from build123d import *

# Parameters (mm, degrees)
F1_DEPTH = 10
F2_R     = 11
F3_DEPTH = 7.5
F4_R     = 4
F5_DEPTH = 7
F6_R     = 5
F7_DEPTH = 25
F8_R     = 2


# Not quite as in the source:
# - a feature names something its author has since deleted; it is built from what else it names


with BuildPart() as f1:
    # F0 (on Top) → F1 (new body)
    with BuildSketch(Plane.XY):
        with BuildLine():
            Line((29.69714, -15), (29.69714, 0))
            ThreePointArc((29.69714, 0), (27.1937406538, 6.0437406538), (21.15, 8.54714))
            Line((21.15, 8.54714), (12.3266539588, 8.54714))
            ThreePointArc((12.3266539588, 8.54714), (0, 15), (-12.3266539588, 8.54714))
            Line((-12.3266539588, 8.54714), (-21.15, 8.54714))
            ThreePointArc((-21.15, 8.54714), (-29.69714, 0), (-21.15, -8.54714))
            Line((-21.15, -8.54714), (-12.3266539588, -8.54714))
            ThreePointArc((-12.3266539588, -8.54714), (-6.9567557094, -13.2892268398), (0, -15))
            Line((0, -15), (29.69714, -15))
        make_face()
    extrude(amount=F1_DEPTH)

    # F2 (on face) → F3 (cut)
    with BuildSketch(Plane.XY.offset(10)):
        Circle(F2_R)
    extrude(amount=-F3_DEPTH, mode=Mode.SUBTRACT)

    # F4 (on face) → F5 (cut)
    with BuildSketch(Plane(origin=(0, 0, 0), x_dir=(1, 0, 0), z_dir=(0, 0, -1))):
        with Locations((-21.15, 0)):
            Circle(F4_R)
        with Locations((21.15, 0)):
            Circle(F4_R)
    extrude(amount=-F5_DEPTH, mode=Mode.SUBTRACT)

    # F6 (on face) → F7 (cut)
    with BuildSketch(Plane.XY.offset(2.5)):
        with Locations((0, 0.6768586167)):
            Circle(F6_R)
    extrude(amount=-F7_DEPTH, mode=Mode.SUBTRACT)

    # F8
    f8_edges = [f1.edges().sort_by_distance(p)[0] for p in [
        (29.69714, -15, 5),
    ]]
    fillet(f8_edges, radius=F8_R)


solid = f1.part
Here's how the part is built. I have some questions about the finished solid (model axes, mm). A direction names the side the tool comes from. Give positions to 0.01 mm unless a question says otherwise; leave off trailing zeros. Write each loop counter-clockwise with the first axis right and the second up, starting at its lowest first coordinate (ties: lowest second). Pieces come first, ordered by that corner, then holes. Notation, with made-up numbers: (59.5, 37.25) -> (75.5, 37.25) arc R3 ccw to (75.5, 41.25) -> close; hole circle Ø10 at (-11, -16). An arc over 180 degrees is marked (long way). Use one line per item in the form item = value. Start each with the question number.
1. Imagine slicing it at D-D on z = 1.75. List the corners of the cut face in (x, y) for me, plus the area to 3 significant figures.
2. If I drill on L1, parallel to X at y = -2.5, z = 5.75; L2, parallel to Y at x = 0, z = 6.75; L3, parallel to X at y = -3, z = 1.25, over which ranges is the centre line in solid material (lowest first)?
3. Thinking about a two-plate mould opening in Y: for faces 1 (the face through (6, 0, 0)), 2 (the face through (-17, -8.547, 5)), 3 (the face through (21, 0, 7)), which applies, +Y half, -Y half, draft (parallel to the pull), parting line (faces both ways), or undercut?
4. Will these pins go through, and if not, where does the flat tip stop? pin 1 Ø10.5 at (x, y) = (-21.15, 0) entering from -Z; pin 2 Ø2.5 at (x, z) = (18, 7) entering from +Y; pin 3 Ø6.5 at (x, y) = (-3, -5) entering from +Z; pin 4 Ø1 at (y, z) = (1, 2) entering from -X.
5. On a 3-axis mill with a long thin cutter (end or side, diameter ignored), from which of +Z, -Z, +X, -X, +Y, -Y can I reach the whole of each face in a straight line? I mean faces 4 (the face through (0, -5, 2.5)), 5 (the face through (-17, 8.547, 5)), 6 (the face through (17, 8.547, 5)), 7 (the face through (17.976, 2.434, 3.451)), 8 (the face through (2.69, 4.89, 1.27)). Say none if no direction works.
6. Imagine slicing it at B-B on x = 24. List the corners of the cut face in (y, z) for me, plus the area to 3 significant figures.
7. Imagine slicing it at A-A on z = 4.5. List the corners of the cut face in (x, y) for me, plus the area to 3 significant figures.
8. Imagine slicing it at C-C on y = -6. List the corners of the cut face in (x, z) for me.
Entries:
q1.outline = (-21.15, -8.55) -> (-12.33, -8.55) arc R15 ccw to (0, -15) -> (27.7, -15) arc R2 ccw to (29.7, -13) -> (29.7, 0) arc R8.55 ccw to (21.15, 8.55) -> (12.33, 8.55) arc R15 ccw to (-12.33, 8.55) -> (-21.15, 8.55) arc R8.55 ccw to start; hole circle Ø8 at (-21.15, 0); hole circle Ø10 at (0, 0.68); hole circle Ø8 at (21.15, 0)
q1.area = 1,150 mm²
q2.L1 = -29.32 to -24.27, -18.03 to -10.71, 10.71 to 18.03, 24.27 to 29.7
q2.L2 = -15 to -11, 11 to 15
q2.L3 = -29.15 to -23.8, -18.5 to -3.39, 3.39 to 18.5, 23.8 to 29.7
q3.face_1 = draft
q3.face_2 = -Y half
q3.face_3 = undercut
q4.pin_1 = 0
q4.pin_2 = 8.55
q4.pin_3 = 2.5
q4.pin_4 = -29.68
q5.face_4 = +Z
q5.face_5 = +Z, -Z, -X, +Y
q5.face_6 = +Z, -Z, +X, +Y
q5.face_7 = -Z
q5.face_8 = +Z, -Z
q6.outline = (-15, 0) -> (-2.81, 0) -> (-2.81, 7) -> (2.81, 7) -> (2.81, 0) -> (8.06, 0) -> (8.06, 10) -> (-15, 10) -> close
q6.area = 191 mm²
q7.outline = (-21.15, -8.55) -> (-12.33, -8.55) arc R15 ccw to (0, -15) -> (27.7, -15) arc R2 ccw to (29.7, -13) -> (29.7, 0) arc R8.55 ccw to (21.15, 8.55) -> (12.33, 8.55) arc R15 ccw to (-12.33, 8.55) -> (-21.15, 8.55) arc R8.55 ccw to start; hole circle Ø8 at (-21.15, 0); hole circle Ø22 at (0, 0); hole circle Ø8 at (21.15, 0)
q7.area = 846 mm²
q8.outline = (-27.24, 0) -> (29.7, 0) -> (29.7, 10) -> (9.22, 10) -> (9.22, 2.5) -> (-9.22, 2.5) -> (-9.22, 10) -> (-27.24, 10) -> close
